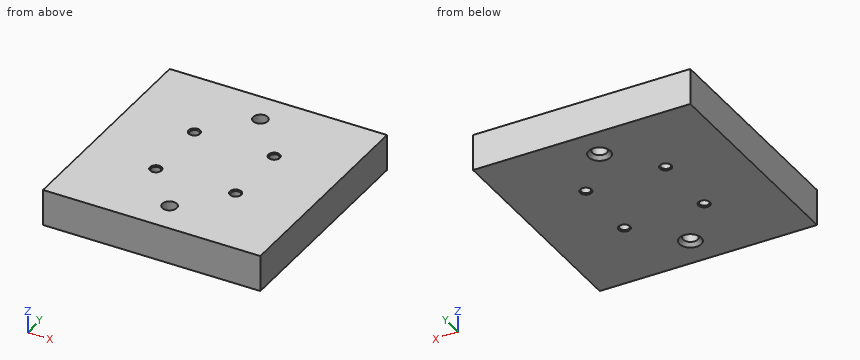
```python
from build123d import *

# Parameters (mm, degrees)
SKETCH1_W                         = 76.2
SKETCH1_H                         = 78.74
BOSS_EXTRUDE1_DEPTH               = 12.7
F_1_4_20_TAPPED_HOLE1_D           = 5.1054
F_1_4_20_TAPPED_HOLE1_CSINK_D     = 7.62
F_1_4_20_TAPPED_HOLE1_CSINK_ANGLE = 90
M4_TAPPED_HOLE1_AT_2_COUNT        = 2
M4_TAPPED_HOLE1_AT_2_PITCH        = 27.9908
M4_TAPPED_HOLE1_AT_3_COUNT        = 2
M4_TAPPED_HOLE1_AT_3_PITCH        = 36.856616589
M4_TAPPED_HOLE1_AT_4_COUNT        = 2
M4_TAPPED_HOLE1_AT_4_PITCH        = 23.9776


with BuildPart() as part:
    # Sketch1 → Boss-Extrude1 (new body)
    with BuildSketch(Plane.XY):
        Rectangle(SKETCH1_W, SKETCH1_H)
    extrude(amount=BOSS_EXTRUDE1_DEPTH)

    # 1/4-20 Tapped Hole1 (through all)
    with Locations(Plane(origin=(0, 0, 0), x_dir=(-1, 0, 0), z_dir=(0, 0, -1))):
        with Locations((0, 28.2321), (0, -28.2321)):
            CounterSinkHole(F_1_4_20_TAPPED_HOLE1_D / 2, F_1_4_20_TAPPED_HOLE1_CSINK_D / 2, counter_sink_angle=F_1_4_20_TAPPED_HOLE1_CSINK_ANGLE)

    # Sketch5 → M4 Tapped Hole1 (revolve, cut)
    with BuildSketch(Plane(origin=(13.9954, 11.9888, 0), x_dir=(0, 1, 0), z_dir=(1, 0, 0))):
        Polygon((0, 0), (0, 12.7), (2.025, 12.7), (1.65, 12.325), (1.65, 0.375), (2.025, 0), align=None)
    m4_tapped_hole1 = revolve(axis=Axis((13.9954, 11.9888, -6.35), (0, 0, 1)), mode=Mode.SUBTRACT)

    # M4 Tapped Hole1 at 2: M4 Tapped Hole1 ×2
    with Locations(*[(-i * M4_TAPPED_HOLE1_AT_2_PITCH, 0, 0) for i in range(1, M4_TAPPED_HOLE1_AT_2_COUNT)]):
        add(m4_tapped_hole1, mode=Mode.SUBTRACT)

    # M4 Tapped Hole1 at 3: M4 Tapped Hole1 ×2
    with Locations(*[Vector(-0.7594511539682676, -0.6505643279002215, 0) * (i * M4_TAPPED_HOLE1_AT_3_PITCH) for i in range(1, M4_TAPPED_HOLE1_AT_3_COUNT)]):
        add(m4_tapped_hole1, mode=Mode.SUBTRACT)

    # M4 Tapped Hole1 at 4: M4 Tapped Hole1 ×2
    with Locations(*[(0, -i * M4_TAPPED_HOLE1_AT_4_PITCH, 0) for i in range(1, M4_TAPPED_HOLE1_AT_4_COUNT)]):
        add(m4_tapped_hole1, mode=Mode.SUBTRACT)


solid = part.part
```
Work out the finished part from the listing and answer in its coordinate system (mm). Coordinates: 2 decimals unless noted, no trailing zeros. Write each loop counter-clockwise with the first axis right and the second up, starting at its lowest first coordinate (ties: lowest second). Pieces come first, ordered by that corner, then holes.
Q1. A cutting plane is placed at A-A, the plane x = 0. Give the vertices of the cut face in (y, z), then the cut area to 3 significant figures.
Q2. Find the intervals of material crossed by line 1 (X direction, y = 12, z = 2); line 2 (Y direction, x = 0, z = 6.75); line 3 (Y direction, x = 12.5, z = 9.25), in increasing order.
Q3. This flat-tipped pin is pushed along its axis until it touches: pin 1 Ø6 at (x, y) = (0, 28.23) entering from -Z. Where does it stop, or does it pass through?
Findings below:
1. outline: (-39.37, 0) - (-32.04, 0) - (-30.78, 1.26) - (-30.78, 12.7) - (-39.37, 12.7) - close; (-25.68, 1.26) - (-24.42, 0) - (24.42, 0) - (25.68, 1.26) - (25.68, 12.7) - (-25.68, 12.7) - close; (30.78, 1.26) - (32.04, 0) - (39.37, 0) - (39.37, 12.7) - (30.78, 12.7) - close
1. area: 867 mm2
2. line 1: x = -38.1 to -15.65, -12.35 to 12.35, 15.65 to 38.1
2. line 2: y = -39.37 to -30.78, -25.68 to 25.68, 30.78 to 39.37
2. line 3: y = -39.37 to -12.69, -11.29 to 11.29, 12.69 to 39.37
3. pin 1: stops at z = 0.81
